Autodesk Inventor part; units mm, degrees
ref_plane "YZ Plane" through (0, 0, 0) normal (1, 0, 0) x (0, 1, 0)
ref_plane "XZ Plane" through (0, 0, 0) normal (0, 1, 0) x (-1, 0, 0)
ref_plane "XY Plane" through (0, 0, 0) normal (0, 0, 1) x (1, 0, 0)
sketch "Sketch1" plane through (0, 0, 0) normal (0, 0, 1) x (1, 0, 0)
  line L0 (0, 0) -> (20, 0)
  line L1 (20, 0) -> (20, 3.2)
  line L2 (0, 3.2) -> (20, 3.2)
  line L3 (0, 0) -> (0, 3.2)
  line L4 (20, -25) -> (0, -25)
  line L5 (0, -25) -> (0, -28.2)
  line L6 (20, -28.2) -> (0, -28.2)
  line L7 (20, -25) -> (20, -28.2)
  line L8 (3.2, -25) -> (3.2, 0)
  line L9 (0, -25) -> (0, 0)
  line L10 (-0.3, -0.3) -> (-0.3, 3.5)
  line L11 (-0.3, 3.5) -> (20.3, 3.5)
  line L12 (20.3, 3.5) -> (20.3, -0.3)
  line L13 (20.3, -24.7) -> (20.3, -28.5)
  line L14 (20.3, -28.5) -> (-0.3, -28.5)
  line L15 (-0.3, -28.5) -> (-0.3, -24.7)
  line L16 (3.5, -24.7) -> (3.5, -0.3)
  line L17 (-0.3, -0.3) -> (-0.3, -24.7)
  line L18 (20.3, -0.3) -> (3.5, -0.3)
  line L19 (3.5, -24.7) -> (20.3, -24.7)
  line L20 (6.5, -3.3) -> (6.5, -21.7)
  line L21 (6.5, -21.7) -> (23.3, -21.7)
  line L22 (23.3, -21.7) -> (23.3, -31.5)
  line L23 (23.3, -31.5) -> (-3.3, -31.5)
  line L24 (-3.3, -31.5) -> (-3.3, -24.7)
  line L25 (-3.3, -24.7) -> (-3.3, -0.3)
  line L26 (-3.3, -0.3) -> (-3.3, 6.5)
  line L27 (-3.3, 6.5) -> (23.3, 6.5)
  line L28 (23.3, 6.5) -> (23.3, -3.3)
  line L29 (23.3, -3.3) -> (6.5, -3.3)
  dimension "d2" = 0.3
  dimension "d3" = 0.3
  dimension "d4" = 0.3
  dimension "d5" = 24.4
  dimension "d6" = 3.8
  dimension "d7" = 3
extrude "Extrusion1" add sketch "Sketch1" against normal blind 15 contours L20 L21 L22 L23 L24 L25 L26 L27 L28 L29
sketch "Sketch4" plane through (0, 0, 0) normal (0, 0, 1) x (1, 0, 0)
  line L0 (23.3, -3.3) -> (23.3, 6.5)
  line L1 (23.3, 6.5) -> (-3.3, 6.5)
  line L2 (23.3, -3.3) -> (6.5, -3.3)
  line L3 (6.5, -3.3) -> (6.5, -21.7)
  line L4 (6.5, -21.7) -> (23.3, -21.7)
  line L5 (-3.3, -0.3) -> (-3.3, 6.5)
  line L6 (-3.3, -31.5) -> (23.3, -31.5)
  line L7 (23.3, -31.5) -> (23.3, -21.7)
  line L8 (23.3, -21.7) -> (6.5, -21.7)
  line L9 (23.3, 6.5) -> (23.3, -3.3)
  line L10 (23.3, -3.3) -> (23.3, 6.5)
  line L11 (-3.3, -31.5) -> (-3.3, 6.5)
  line L12 (23.3, 6.5) -> (-3.3, 6.5)
  line L13 (-3.3, 6.5) -> (-3.3, -31.5)
  line L14 (23.3, -31.5) -> (-3.3, -31.5)
  line L15 (-3.3, -31.5) -> (23.3, -31.5)
  line L16 (23.3, -21.7) -> (23.3, -31.5)
  line L17 (23.3, -31.5) -> (23.3, -21.7)
  line L18 (6.5, -3.3) -> (6.5, -21.7)
  line L19 (23.3, -3.3) -> (6.5, -3.3)
  line L20 (6.5, -3.3) -> (23.3, -3.3)
  line L21 (23.3, -3.3) -> (23.3, -21.7)
  point P0 (0, 0)
extrude "Extrusion3" add sketch "Sketch4" along normal blind 3
sketch "Sketch5" plane through (6.5, -21.7, -15) normal (1, 0, 0) x (0, 0, -1)
  line L0 (0, 18.4) -> (0, 0)
  line L1 (-15, 18.4) -> (0, 18.4)
  line L2 (-15, 0) -> (0, 0)
  line L3 (-15, 0) -> (-15, 18.4)
  circle A0 centre (-6, 9.2) radius 2
  circle A1 centre (-6, 9.2) radius 4
  point P0 (-15, 21.7)
  dimension "d14" = 4
  dimension "d15" = 6
  dimension "d16" = 8
  dimension "d17" = 9.2
extrude "Extrusion4" cut sketch "Sketch5" against normal blind 1 contours A1
extrude "Extrusion5" cut sketch "Sketch5" against normal blind 80 contours A0
properties part number "Tope_Carril"
Here's how the part is built. I have some questions about the finished solid (model axes, mm). A direction names the side the tool comes from. Round coordinates to 2 decimals unless told otherwise and drop trailing zeros. Write each loop counter-clockwise with the first axis right and the second up, starting at its lowest first coordinate (ties: lowest second). Pieces come first, ordered by that corner, then holes.
1. For faces 4 (the flat face through (10, -28.5, -7)), 5 (the cylindrical face through (6.007, -12.324, -5.004)), 6 (the flat face through (15, -21.7, -7)), which set-ups out of +Z, -Z, +X, -X, +Y, -Y let a thin tool reach every point of the face, with its end or its side?
2. If we mould it in two halves opening along Y, with no side actions, what happens to faces 1 (the flat face through (3.5, -13, -6)), 2 (the flat face through (10, 6.5, -6)), 3 (the flat face through (10, -12, 3))? For each: released by +Y, released by -Y, zero draft, split by the parting line, or undercut.
3. Will these pins go through, and if not, where does the flat tip stop? pin 1 Ø5 at (y, z) = (-12.5, -9) entering from +X; pin 2 Ø6.5 at (y, z) = (-13, -10.5) entering from +X.
4. Suppose I cut it at D-D (x = 2.5). List the corners of the cut face in (y, z) for me, and give its area (3 significant figures).
5. Suppose I cut it at B-B (z = -2.75). List the corners of the cut face in (x, y) for me.
6. I need wall thicknesses on L1, parallel to Y at x = 4.5, z = -9; L2, parallel to Y at x = 4.25, z = -1.75; L3, parallel to Y at x = 8.25, z = -5.25. Which ranges of each line are inside material? Lowest first, please.
7. Suppose I cut it at A-A (y = -12.5). List the corners of the cut face in (x, z) for me.
8. Suppose I cut it at C-C (z = -9). List the corners of the cut face in (x, y) for me, and give its area (3 significant figures).
Answer sheet:
1. face 4: -Z
1. face 5: +X
1. face 6: -Z, +X
2. face 1: undercut
2. face 2: released by +Y
2. face 3: zero draft
3. pin 1: stops at x = 5.5
3. pin 2: stops at x = 6.5
4. outline: (-31.5, -15) - (-28.5, -15) - (-28.5, 0) - (3.5, 0) - (3.5, -15) - (6.5, -15) - (6.5, 3) - (-31.5, 3) - close
4. area: 204 mm2
5. outline: (-3.3, -31.5) - (23.3, -31.5) - (23.3, -21.7) - (6.5, -21.7) - (6.5, -3.3) - (23.3, -3.3) - (23.3, 6.5) - (-3.3, 6.5) - close; hole (-0.3, -28.5) - (20.3, -28.5) - (20.3, -24.7) - (3.5, -24.7) - (3.5, -0.3) - (20.3, -0.3) - (20.3, 3.5) - (-0.3, 3.5) - close
6. L1: y = -31.5 to -28.5, -24.7 to -14.5, -10.5 to -0.3, 3.5 to 6.5
6. L2: y = -31.5 to -28.5, -24.7 to -0.3, 3.5 to 6.5
6. L3: y = -31.5 to -28.5, -24.7 to -21.7, -3.3 to -0.3, 3.5 to 6.5
7. outline: (-3.3, -15) - (-0.3, -15) - (-0.3, -11) - (-3.3, -11) - close; (-3.3, -7) - (-0.3, -7) - (-0.3, 0) - (3.5, 0) - (3.5, -7) - (5.5, -7) - (5.5, -5) - (6.5, -5) - (6.5, 0) - (23.3, 0) - (23.3, 3) - (-3.3, 3) - close; (3.5, -15) - (6.5, -15) - (6.5, -13) - (5.5, -13) - (5.5, -11) - (3.5, -11) - close
8. outline: (-3.3, -31.5) - (23.3, -31.5) - (23.3, -21.7) - (6.5, -21.7) - (6.5, -16.5) - (5.5, -16.5) - (5.5, -14.5) - (3.5, -14.5) - (3.5, -24.7) - (20.3, -24.7) - (20.3, -28.5) - (-0.3, -28.5) - (-0.3, -14.5) - (-3.3, -14.5) - close; (-3.3, -10.5) - (-0.3, -10.5) - (-0.3, 3.5) - (20.3, 3.5) - (20.3, -0.3) - (3.5, -0.3) - (3.5, -10.5) - (5.5, -10.5) - (5.5, -8.5) - (6.5, -8.5) - (6.5, -3.3) - (23.3, -3.3) - (23.3, 6.5) - (-3.3, 6.5) - close
8. area: 424 mm2
